```python
from build123d import *

# Parameters (mm, degrees)
BOSS_EXTRUDE1_DEPTH     = 25.5
SKETCH2_R               = 4.5
CUT_EXTRUDE1_DEPTH      = 25
SKETCH3_R               = 1.5
CUT_EXTRUDE2_DEPTH      = 10
SKETCH4_R               = 5
CUT_EXTRUDE3_DEPTH      = 2
CUT_EXTRUDE4_DEPTH      = 3
CUT_EXTRUDE5_DEPTH      = 3
SKETCH7_R               = 4.5
CUT_EXTRUDE6_DEPTH      = 2
CUT_EXTRUDE7_DEPTH      = 108.685885798
CUT_EXTRUDE7_DEPTH_BACK = 108.685885798
SKETCH8_R               = 1.5
CUT_EXTRUDE8_START      = -10
SKETCH9_R               = 4.5
CUT_EXTRUDE8_DEPTH      = 10
BOSS_EXTRUDE2_DEPTH     = 25.5
SKETCH11_W              = 20
SKETCH11_H              = 20
BOSS_EXTRUDE3_DEPTH     = 2


with BuildPart() as part:
    # Sketch1 → Boss-Extrude1 (new body)
    with BuildSketch(Plane(origin=(0, 0, 0), x_dir=(1, 0, 0), z_dir=(0, 1, 0))):
        Polygon((6, -6), (55, -6), (55, -85), (61, -85), (61, 60), (55, 60), (55, 0), (6, 0), (6, 60), (0, 60), (0, -85), (6, -85), align=None)
    extrude(amount=BOSS_EXTRUDE1_DEPTH)

    # Sketch2 → Cut-Extrude1 (cut)
    with BuildSketch(Plane(origin=(6, 0, 0), x_dir=(0, 0, -1), z_dir=(1, 0, 0))):
        with Locations((-71, 12.75)):
            Circle(SKETCH2_R)
    extrude(amount=-CUT_EXTRUDE1_DEPTH, mode=Mode.SUBTRACT)

    # Sketch3 → Cut-Extrude2 (cut)
    with BuildSketch(Plane.ZY.offset(-55)):
        with Locations((71, 12.75)):
            Circle(SKETCH3_R)
    extrude(amount=-CUT_EXTRUDE2_DEPTH, mode=Mode.SUBTRACT)

    # Sketch4 → Cut-Extrude3 (cut)
    with BuildSketch(Plane(origin=(61, 0, 0), x_dir=(0, 0, -1), z_dir=(1, 0, 0))):
        with Locations((-71, 12.75)):
            Circle(SKETCH4_R)
    extrude(amount=-CUT_EXTRUDE3_DEPTH, mode=Mode.SUBTRACT)

    # Sketch5 → Cut-Extrude4 (cut)
    with BuildSketch(Plane.ZY.offset(-55)):
        with BuildLine():
            Line((71, 19.25), (54, 15.75))
            ThreePointArc((54, 15.75), (51, 12.75), (54, 9.75))
            Line((54, 9.75), (71, 6.25))
            ThreePointArc((71, 6.25), (77.5, 12.75), (71, 19.25))
        make_face()
    extrude(amount=-CUT_EXTRUDE4_DEPTH, mode=Mode.SUBTRACT)

    # Sketch6 → Cut-Extrude5 (cut)
    with BuildSketch(Plane.ZY.offset(-55)):
        with BuildLine():
            Line((-29, 9.75), (-46, 6.25))
            ThreePointArc((-46, 6.25), (-52.5, 12.75), (-46, 19.25))
            Line((-46, 19.25), (-29, 15.75))
            ThreePointArc((-29, 15.75), (-26, 12.75), (-29, 9.75))
        make_face()
    extrude(amount=-CUT_EXTRUDE5_DEPTH, mode=Mode.SUBTRACT)

    # Sketch7 → Cut-Extrude6 (cut)
    with BuildSketch(Plane(origin=(61, 0, 0), x_dir=(0, 0, -1), z_dir=(1, 0, 0))):
        with Locations((46, 12.75)):
            Circle(SKETCH7_R)
    extrude(amount=-CUT_EXTRUDE6_DEPTH, mode=Mode.SUBTRACT)

    # Sketch8 → Cut-Extrude7 (cut, two sides: drawn at the far end of the back side and taken through both)
    with BuildSketch(Plane(origin=(61, 0, 0), x_dir=(0, 0, -1), z_dir=(1, 0, 0)).offset(-CUT_EXTRUDE7_DEPTH_BACK)):
        with Locations((46, 12.75)):
            Circle(SKETCH8_R)
    extrude(amount=CUT_EXTRUDE7_DEPTH + CUT_EXTRUDE7_DEPTH_BACK, mode=Mode.SUBTRACT)

    # Sketch9 → Cut-Extrude8 (cut)
    with BuildSketch(Plane.ZY.offset(CUT_EXTRUDE8_START)):
        with Locations(Location((-46, 12.75, 0), (0, 0, 180))):
            Circle(SKETCH9_R)
    extrude(amount=CUT_EXTRUDE8_DEPTH, mode=Mode.SUBTRACT)

    # Sketch10 → Boss-Extrude2 (add)
    with BuildSketch(Plane(origin=(0, 25.5, 0), x_dir=(1, 0, 0), z_dir=(0, 1, 0))):
        Polygon((9, -6), (6, -6), (6, -9), align=None)
        Polygon((6, 0), (6, 3), (9, 0), align=None)
        Polygon((52, 0), (55, 0), (55, 3), align=None)
        Polygon((55, -6), (55, -9), (52, -6), align=None)
    extrude(amount=-BOSS_EXTRUDE2_DEPTH)

    # Sketch11 → Boss-Extrude3 (add)
    with BuildSketch(Plane.XZ):
        with Locations((3, -56)):
            Rectangle(SKETCH11_W, SKETCH11_H)
        with Locations((3, 81)):
            Rectangle(SKETCH11_W, SKETCH11_H)
        with Locations((58, 81)):
            Rectangle(SKETCH11_W, SKETCH11_H)
        with Locations((58, -56)):
            Rectangle(SKETCH11_W, SKETCH11_H)
    extrude(amount=-BOSS_EXTRUDE3_DEPTH)


solid = part.part
```
Could you check a few things on this model? Use its own coordinates, in mm. A direction names the side the tool comes from. Round coordinates to 2 decimals unless told otherwise and drop trailing zeros. Loops run counter-clockwise (first coordinate to the right, second up) from the corner with the lowest first, then second, coordinate; pieces in that order, holes last. Notation, with made-up numbers: (-19, 32) - (30, 32) arc R21 ccw to (30, 55) - close; hole circle Ø2 at (65, 20.5). An arc over 180 degrees is marked (long way). Answer in a Markdown table with one row per item. Add a question column.
(1) I need wall thicknesses on line 1 along X through (y, z) = (9.25, 25); line 2 along Y through (x, z) = (58.6, 71); line 3 along Y through (x, z) = (3.3, -46). Which ranges of each line are inside material? Lowest first, please.
(2) If we mould it in two halves opening along Z, with no side actions, what happens to faces 1 (the face through (58, 14, -60)), 2 (the face through (56.479, 8.024, 62.381)), 3 (the face through (57.9, 2, -60.3)), 4 (the face through (56.479, 17.524, 62.619))? For each: pulls with the +Z half, pulls with the -Z half, needs draft (parallel to the pull), parting line crosses it, or undercut.
(3) If we section it at A-A (z = 35.5): Please give me the cut outline in (x, y), plus the area to 3 significant figures.
(4) I'm going to push flat-ended pins straight in: pin 1 (11.5 mm diameter, centred on y = 12.75, z = -46, fed in from -X); pin 2 (8 mm diameter, centred on x = 39.5, y = 17, fed in from -Z); pin 3 (10 mm diameter, centred on x = 32, y = 8.5, fed in from +Z); pin 4 (10 mm diameter, centred on x = 49.5, z = 57, fed in from +Y). Where does each tip first touch, or does it pass through?
(5) If we section it at D-D (z = -38.5): Please give me the cut outline in (x, y), plus the area to 3 significant figures.
(6) For faces 5 (the face through (3, 14, -60)), 6 (the face through (60.014, 14.102, -50.292)), 7 (the face through (58.5, 12.8, -44.5)), 8 (the face through (58, 13, 67)), which set-ups out of +Z, -Z, +X, -X, +Y, -Y let a thin tool reach every point of the face, with its end or its side?
(7) If we section it at C-C (y = 12.75): State how many separate pieces and enclosed holes the cut face has, plus the area to 3 significant figures.
(8) If we section it at B-B (y = 21.75): Please give me the cut outline in (x, z), plus the area to 3 significant figures.
Model answer:
| question | item | result |
|---|---|---|
| 1 | line 1 | x = 0 to 6, 55 to 61 |
| 1 | line 2 | y = 0 to 11.25, 14.25 to 25.5 |
| 1 | line 3 | y = 0 to 8.25, 17.25 to 25.5 |
| 2 | face 1 | pulls with the -Z half |
| 2 | face 2 | undercut |
| 2 | face 3 | needs draft |
| 2 | face 4 | undercut |
| 3 | outline | (0, 0) - (6, 0) - (6, 25.5) - (0, 25.5) - close; (55, 0) - (61, 0) - (61, 25.5) - (55, 25.5) - close |
| 3 | area | 306 mm² |
| 4 | pin 1 | stops at x = 0 |
| 4 | pin 2 | stops at z = 0 |
| 4 | pin 3 | stops at z = 6 |
| 4 | pin 4 | passes through |
| 5 | outline | (0, 0) - (6, 0) - (6, 25.5) - (0, 25.5) - close; (55, 0) - (61, 0) - (61, 25.5) - (55, 25.5) - (55, 17.71) - (58, 17.71) - (58, 7.79) - (55, 7.79) - close |
| 5 | area | 276 mm² |
| 6 | face 5 | -Z, +X, -X, +Y |
| 6 | face 6 | +X |
| 6 | face 7 | +X, -X |
| 6 | face 8 | none |
| 7 | separate pieces | 5 |
| 7 | enclosed holes | 0 |
| 7 | area | 1,740 mm² |
| 8 | outline | (0, -60) - (6, -60) - (6, -3) - (9, 0) - (52, 0) - (55, -3) - (55, -60) - (61, -60) - (61, 85) - (55, 85) - (55, 9) - (52, 6) - (9, 6) - (6, 9) - (6, 85) - (0, 85) - close |
| 8 | area | 2,050 mm² |
